```python
from build123d import *

# Parameters (mm, degrees)
SKETCH2_R          = 1.5
CUT_EXTRUDE1_DEPTH = 14


with BuildPart() as part:
    # Sketch1 → Revolve1 (revolve)
    with BuildSketch(Plane.XY):
        Polygon((55, 0), (63, 10), (66.841874542, 10), (56.441874542, -3), (0, -3), (0, 0), align=None)
    revolve(axis=Axis((0, -3, 0), (0, 1, 0)))

    # Sketch2 → Cut-Extrude1 (cut, through all)
    with BuildSketch(Plane(origin=(0, -3, 0), x_dir=(-1, 0, 0), z_dir=(0, -1, 0))):
        with Locations((0, -27.5)):
            Circle(SKETCH2_R)
        with Locations((-19.445436483, -19.445436483)):
            Circle(SKETCH2_R)
        with Locations((-27.5, 0)):
            Circle(SKETCH2_R)
        with Locations((-19.445436483, 19.445436483)):
            Circle(SKETCH2_R)
        with Locations((0, 27.5)):
            Circle(SKETCH2_R)
        with Locations((19.445436483, 19.445436483)):
            Circle(SKETCH2_R)
        with Locations((27.5, 0)):
            Circle(SKETCH2_R)
        with Locations((19.445436483, -19.445436483)):
            Circle(SKETCH2_R)
    extrude(amount=-CUT_EXTRUDE1_DEPTH, mode=Mode.SUBTRACT)


solid = part.part
```
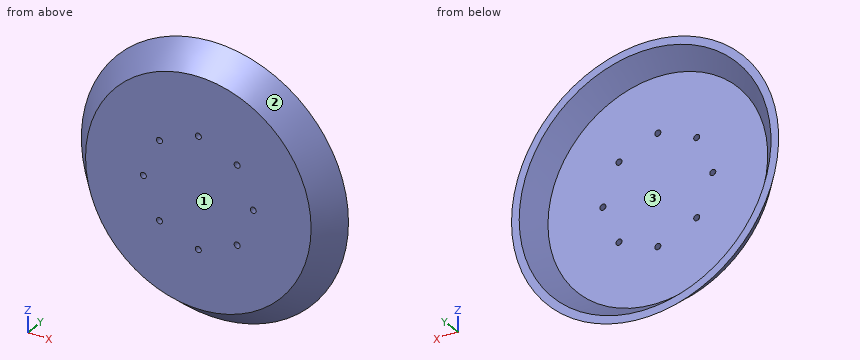
Part model, mm, in its own coordinate system. Face numbers are marked on the shaded views. Round coordinates to 2 decimals unless told otherwise and drop trailing zeros. Loops run counter-clockwise (first coordinate to the right, second up) from the corner with the lowest first, then second, coordinate; pieces in that order, holes last.
1. Two-plate mould, pull along X, no slides. Class the marked faces 1, 2 and 3: pulls with the +X half, pulls with the -X half, needs draft (parallel to the pull), parting line crosses it, or undercut.
Solutions:
face 1: needs draft
face 2: parting line crosses it
face 3: undercut
2. Flat gauge pins, fed straight in: pin 1 (5 mm diameter, centred on x = 27.5, z = 0, fed in from +Y); pin 2 (3 mm diameter, centred on y = 2, z = -45, fed in from +X); pin 3 (3 mm diameter, centred on y = -0.5, z = 42.5, fed in from +X). Where does each tip first touch, or does it go through?
Solutions:
pin 1: stops at y = 0
pin 2: stops at x = 42.73
pin 3: stops at x = 42.41
3. Slice it at A-A (y = 5). Give the cut face in (x, z), and give its area (3 significant figures).
Solutions:
outline: circle Ø125.68 at (0, 0); hole circle Ø118 at (0, 0)
area: 1,470 mm2
4. Drill centre lines: line 1 along Z through (x, y) = (0, -1.1); line 2 along Z through (x, y) = (0, -1.4); line 3 along Y through (x, z) = (-17.5, 13). Where is each one in solid material? Low to high.
Solutions:
line 1: z = -57.96 to -29, -26 to 26, 29 to 57.96
line 2: z = -57.72 to -29, -26 to 26, 29 to 57.72
line 3: y = -3 to 0
